Input: part model. Units: mm. Frame: model coordinates. Face numbers are marked on the shaded views. Coordinates: 2 decimals unless noted, no trailing zeros. Loops run counter-clockwise (first coordinate to the right, second up) from the corner with the lowest first, then second, coordinate; pieces in that order, holes last. Notation, with made-up numbers: M 89,26 L 121,26 A10 ccw 121,40 Z; hole C 67,44 d9. An arc over 180 degrees is marked long. Use a Markdown table: item, result. Add a question column.
1. Section C-C on x = -3. Output: boundary loops of the cut face in (y, z).
2. Pin query (flat end, axial travel): pin 1 (0.5 mm diameter, centred on y = 0.5, z = 0, fed in from +X); pin 2 (0.9 mm diameter, centred on y = 0, z = -0.5, fed in from +X). Return the tip coordinate at first contact, or that it passes through.
3. Draft query along Z for the marked faces 1, 2 and 3. Return one class per face: +Z half, -Z half, draft (parallel to the pull), parting line (faces both ways), or undercut.
4. Section D-D on y = -0.5. State how many separate pieces and enclosed holes the cut face has, then the cut area to 3 significant figures.
5. Section B-B on y = -2.45. Output: boundary loops of the cut face in (x, z), then the cut area to 3 significant figures.
6. Line query: L1, parallel to Y at x = -5, z = -0.05; L2, parallel to X at y = 0.5, z = -0.3; L3, parallel to Y at x = -5, z = 0.55. Output: solid intervals per line, ascending. Write a range as [from, to].
```python
from build123d import *

# Parameters (mm, degrees)
SKETCH_1_R          = 1
EXTRUDE_1_DEPTH     = 6
SKETCH_2_R          = 0.9
CUT_EXTRUDE_1_DEPTH = 5.8
SKETCH_5_R          = 0.9
EXTRUDE_4_DEPTH     = 5.6
SKETCH_7_R          = 0.14
FILLET_1_R          = 0.1
FILLET_2_R          = 0.1


with BuildPart() as part:
    # Sketch 1 → Extrude 1 (new body)
    with BuildSketch(Plane(origin=(0, 0, 0), x_dir=(0, 0, -1), z_dir=(1, 0, 0))):
        Circle(SKETCH_1_R)
    extrude(amount=-EXTRUDE_1_DEPTH)

    # Sketch 2 → Cut-Extrude 1 (cut)
    with BuildSketch(Plane(origin=(0, 0, 0), x_dir=(0, 0, -1), z_dir=(1, 0, 0))):
        Circle(SKETCH_2_R)
    extrude(amount=-CUT_EXTRUDE_1_DEPTH, mode=Mode.SUBTRACT)



with BuildPart() as body_2:
    # Sketch 5 → Extrude 4 (new body)
    with BuildSketch(Plane(origin=(-5.8, 0, 0), x_dir=(0, 0, -1), z_dir=(1, 0, 0))):
        Circle(SKETCH_5_R)
    extrude(amount=EXTRUDE_4_DEPTH)


with BuildPart() as part_1:
    add(part.part)

    add(body_2.part)  # Sweep 1 merges body 2
    # Sweep 1: sweep along a curve in space
    with BuildLine() as sweep_1_path:
        Line((-0.2, 0, -0.35), (0, 0, -0.35))
        ThreePointArc((0, 0, -0.35), (0.707106781, -0.292893219, -0.35), (1, -1, -0.35))
        Line((1, -1, -0.35), (1, -3, -0.35))
    # Sketch 7 → Sweep 1 (sweep)
    with BuildSketch(Plane(origin=(-0.2, 0, 0), x_dir=(0, 0, -1), z_dir=(1, 0, 0))):
        with Locations((0.35, 0)):
            Circle(SKETCH_7_R)
    sweep_1 = sweep(path=sweep_1_path.line)

    # Mirror 1: Sweep 1 across plane
    add(sweep_1.mirror(Plane.XY))

    # Fillet 1
    fillet_1_edges = [part_1.edges().sort_by_distance(p)[0] for p in [
        (-6, 0, 1),
    ]]
    fillet(fillet_1_edges, radius=FILLET_1_R)

    # Fillet 2
    fillet_2_edges = [part_1.edges().sort_by_distance(p)[0] for p in [
        (0, 0, 1),
    ]]
    fillet(fillet_2_edges, radius=FILLET_2_R - 0.0001)  # a hair under: the kernel refuses the full size


solid = part_1.part
```
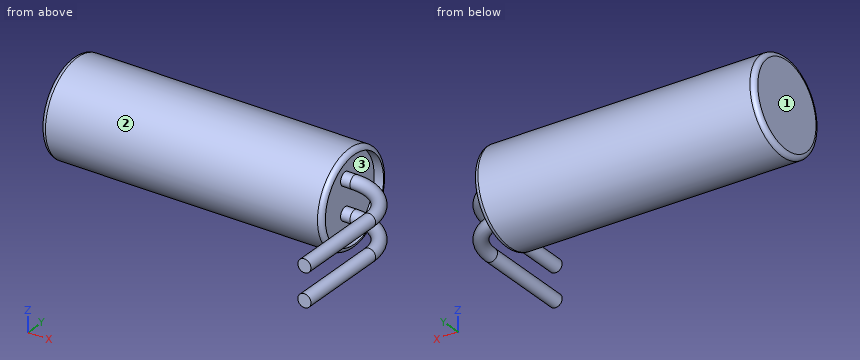
Answers below:
| question | item | result |
|---|---|---|
| 1 | outline | C 0,0 d2 |
| 2 | pin 1 | stops at x = -0.2 |
| 2 | pin 2 | stops at x = 0.99 |
| 3 | face 1 | draft |
| 3 | face 2 | parting line |
| 3 | face 3 | undercut |
| 4 | separate pieces | 3 |
| 4 | enclosed holes | 0 |
| 4 | area | 10.2 mm² |
| 5 | outline | C 1,-0.35 d0.28; C 1,0.35 d0.28 |
| 5 | area | 0.123 mm² |
| 6 | L1 | y = [-1, 1] |
| 6 | L2 | x = [-6, -0.2] |
| 6 | L3 | y = [-0.84, 0.84] |
